```python
from build123d import *

# Parameters (mm, degrees)
SKETCH1_W                = 30.48
SKETCH1_H                = 40.64
INITIAL_BLOCK_DEPTH      = 19.05
INITIAL_BLOCK_DEPTH_BACK = 1.778
SKETCH2_W                = 27.432
SKETCH2_H                = 19.558
INITIAL_CUT_DEPTH        = 38.1
SKETCH20_W               = 5.08
SKETCH20_H               = 10.16
SKETCH20_W_2             = 10.16
SKETCH20_H_2             = 5.08
BOSS_EXTRUDE1_DEPTH      = 1.524
SKETCH21_W               = 2.032
SKETCH21_H               = 24.13
BOSS_EXTRUDE2_DEPTH      = 2.54
SKETCH27_W               = 11.938
SKETCH27_H               = 2.032
CUT_EXTRUDE6_DEPTH       = 1.524
SKETCH28_W               = 30.48
SKETCH28_H               = 1.778
CUT_EXTRUDE7_DEPTH       = 21.828
SKETCH29_W               = 30.48
SKETCH29_H               = 2
CUT_EXTRUDE8_DEPTH       = 6


with BuildPart() as part:
    # Sketch1 → Initial Block (new body, two sides)
    with BuildSketch(Plane.XY) as initial_block_sk:
        with Locations((0, -5.08)):
            Rectangle(SKETCH1_W, SKETCH1_H)
    extrude(amount=INITIAL_BLOCK_DEPTH)
    extrude(initial_block_sk.sketch, amount=-INITIAL_BLOCK_DEPTH_BACK)

    # Sketch2 → Initial Cut (cut)
    with BuildSketch(Plane(origin=(0, 15.24, 0), x_dir=(1, 0, 0), z_dir=(0, 1, 0))):
        with Locations((0, -9.271)):
            Rectangle(SKETCH2_W, SKETCH2_H)
    extrude(amount=-INITIAL_CUT_DEPTH, mode=Mode.SUBTRACT)

    # Sketch20 → Boss-Extrude1 (add)
    with BuildSketch(Plane.XY.offset(19.05)):
        with Locations((-12.7, -6.731)):
            Rectangle(SKETCH20_W, SKETCH20_H)
        with Locations((12.7, -6.731)):
            Rectangle(SKETCH20_W, SKETCH20_H)
        with Locations((0, -20.32)):
            Rectangle(SKETCH20_W_2, SKETCH20_H_2)
    extrude(amount=-BOSS_EXTRUDE1_DEPTH)

    # Sketch21 → Boss-Extrude2 (add)
    with BuildSketch(Plane(origin=(-13.716, 0, 0), x_dir=(0, 0, -1), z_dir=(1, 0, 0))):
        with Locations((-3.556, -10.795)):
            Rectangle(SKETCH21_W, SKETCH21_H)
    boss_extrude2 = extrude(amount=BOSS_EXTRUDE2_DEPTH)

    # Mirror2: Boss-Extrude2 across plane
    add(boss_extrude2.mirror(Plane(origin=(0, 0, 0), x_dir=(0, 0, 1), z_dir=(1, 0, 0))))

    # Sketch27 → Cut-Extrude6 (cut)
    with BuildSketch(Plane(origin=(15.24, 0, 0), x_dir=(0, 0, -1), z_dir=(1, 0, 0))):
        with Locations((-10.795, 8.636)):
            Rectangle(SKETCH27_W, SKETCH27_H)
    cut_extrude6 = extrude(amount=-CUT_EXTRUDE6_DEPTH, mode=Mode.SUBTRACT)

    # Mirror6: Cut-Extrude6 across plane
    add(cut_extrude6.mirror(Plane(origin=(0, 0, 0), x_dir=(0, 0, 1), z_dir=(1, 0, 0))), mode=Mode.SUBTRACT)

    # Sketch28 → Cut-Extrude7 (cut, through all)
    with BuildSketch(Plane.XY.offset(19.05)):
        with Locations((0, 14.351)):
            Rectangle(SKETCH28_W, SKETCH28_H)
    extrude(amount=-CUT_EXTRUDE7_DEPTH, mode=Mode.SUBTRACT)

    # Sketch29 → Cut-Extrude8 (cut)
    with BuildSketch(Plane.XY.offset(19.05)):
        with Locations((0, 12.462)):
            Rectangle(SKETCH29_W, SKETCH29_H)
    extrude(amount=-CUT_EXTRUDE8_DEPTH, mode=Mode.SUBTRACT)


solid = part.part
```
Geometry: final body of the model. Coordinates: model frame, mm. A direction names the side the tool comes from. Round coordinates to 2 decimals unless told otherwise and drop trailing zeros. Order: outer loops, then holes, each group sorted by start corner. A loop starts at its lowest first (then second) coordinate and runs counter-clockwise, first axis right, second up. Notation, with made-up numbers: M 54,33 L 100,33 A34 ccw 100,67 Z; hole C 11,-14 d8. An arc over 180 degrees is marked long. One line per item, written item: value.
(1) Cut plane A-A (z = 7). Return the cut outline in (x, y).
Result sheet:
outline: M -15.24,-25.4 L 15.24,-25.4 L 15.24,7.62 L 13.72,7.62 L 13.72,-22.86 L -13.72,-22.86 L -13.72,7.62 L -15.24,7.62 Z; M -15.24,9.65 L -13.72,9.65 L -13.72,13.46 L -15.24,13.46 Z; M 13.72,9.65 L 15.24,9.65 L 15.24,13.46 L 13.72,13.46 Z
(2) Pin query (flat end, axial travel): P1, Ø1.7, axis at x = 0, z = 18, coming from the +Y side; P2, Ø6, axis at x = 6, z = 10, coming from the +Y side; P3, Ø10, axis at x = 3.5, y = -6.5, coming from the +Z side. Return the tip coordinate at first contact, or that it passes through.
Result sheet:
P1: y = -17.78
P2: y = -22.86
P3: z = -0.51
(3) Pull-direction query (Y, two-part tool) for faces 1 (the flat face through (14, 12, 13.05)), 2 (the flat face through (0, 13.462, -1)), 3 (the flat face through (-14, 9, 4.826)), 4 (the flat face through (-14, 9, 16.764)); classes: pulls with the +Y half, pulls with the -Y half, needs draft (parallel to the pull), parting line crosses it, or undercut.
Result sheet:
face 1: needs draft
face 2: pulls with the +Y half
face 3: undercut
face 4: undercut
(4) Reachability of faces 5 (the flat face through (0, -20, 17.526)), 6 (the flat face through (14, 9, 4.826)), 7 (the flat face through (5.08, -20, 18)) from +Z, -Z, +X, -X, +Y, -Y: full face, straight path, thin tool, end or side. Return the list, or none.
Result sheet:
face 5: +Y
face 6: +X, -X
face 7: +Z, +Y
(5) Cut plane D-D (z = 3.5). Return the cut outline in (x, y).
Result sheet:
outline: M -15.24,-25.4 L 15.24,-25.4 L 15.24,13.46 L 13.72,13.46 L 13.72,1.27 L 11.18,1.27 L 11.18,-22.86 L -11.18,-22.86 L -11.18,1.27 L -13.72,1.27 L -13.72,13.46 L -15.24,13.46 Z
(6) Line query: probe 1 along Z at (x, y) = (12, -4); probe 2 along X at (y, z) = (5.5, 5.75); probe 3 along Y at (x, z) = (-14, 10.5). Output: solid intervals per line, ascending. Write a range as [from, to].
Result sheet:
probe 1: [-1.78, -0.51], [2.54, 4.57], [17.53, 19.05]
probe 2: [-15.24, -13.72], [13.72, 15.24]
probe 3: [-25.4, 7.62], [9.65, 13.46]
(7) Cut plane B-B (y = -1). Return the cut outline in (x, z), and give its area (3 significant figures).
Result sheet:
outline: M -15.24,-1.78 L 15.24,-1.78 L 15.24,19.05 L 13.72,19.05 L 13.72,4.57 L 11.18,4.57 L 11.18,2.54 L 13.72,2.54 L 13.72,-0.51 L -13.72,-0.51 L -13.72,2.54 L -11.18,2.54 L -11.18,4.57 L -13.72,4.57 L -13.72,19.05 L -15.24,19.05 Z
area: 109 mm2
(8) Cut plane C-C (x = -12). Return the cut outline in (y, z), and give its area (3 significant figures).
Result sheet:
outline: M -25.4,-1.78 L 13.46,-1.78 L 13.46,-0.51 L -22.86,-0.51 L -22.86,2.54 L 1.27,2.54 L 1.27,4.57 L -22.86,4.57 L -22.86,19.05 L -25.4,19.05 Z; M -11.81,17.53 L -1.65,17.53 L -1.65,19.05 L -11.81,19.05 Z
area: 164 mm2
